from build123d import *

# Parameters (mm, degrees)
SKETCH_1_W          = 15
SKETCH_1_H          = 15.5
SKETCH_1_R          = 2.55
SKETCH_1_R_2        = 3.05
EXTRUDE_1_DEPTH     = 2.5
CUT_EXTRUDE_START   = 2.5
SKETCH_1_4_R        = 0.9
CUT_EXTRUDE_2_DEPTH = 1
SKETCH_1_5_R        = 0.7
CUT_EXTRUDE_3_DEPTH = 14.747221879


with BuildPart() as part:
    # 草图1 → 凸台-拉伸1 (new body)
    with BuildSketch(Plane(origin=(0, 0, 0), x_dir=(1, 0, 0), z_dir=(0, 1, 0))):
        with Locations((0, -0.25)):
            Rectangle(SKETCH_1_W, SKETCH_1_H)
        with Locations(Location((0, -4.7, 0), (0, 0, 270))):
            Circle(SKETCH_1_R, mode=Mode.SUBTRACT)
        with Locations(Location((0, 3.7, 0), (0, 0, 270))):
            Circle(SKETCH_1_R_2, mode=Mode.SUBTRACT)
    extrude(amount=EXTRUDE_1_DEPTH)

    # 草图1<4> → 切除-拉伸2 (cut)
    with BuildSketch(Plane(origin=(0, 0, 0), x_dir=(1, 0, 0), z_dir=(0, 1, 0)).offset(CUT_EXTRUDE_START)):
        with Locations(Location((-6, -6.5, 0), (0, 0, 90))):
            Circle(SKETCH_1_4_R)
        with Locations(Location((6, 3.5, 0), (0, 0, 90))):
            Circle(SKETCH_1_4_R)
        with Locations(Location((-6, 3.5, 0), (0, 0, 90))):
            Circle(SKETCH_1_4_R)
        with Locations(Location((6, -6.5, 0), (0, 0, 90))):
            Circle(SKETCH_1_4_R)
    extrude(amount=-CUT_EXTRUDE_2_DEPTH, mode=Mode.SUBTRACT)

    # 草图1<5> → 切除-拉伸3 (cut, through all)
    with BuildSketch(Plane(origin=(0, 0, 0), x_dir=(1, 0, 0), z_dir=(0, 1, 0)).offset(CUT_EXTRUDE_START)):
        with Locations(Location((-6, -6.5, 0), (0, 0, 90))):
            Circle(SKETCH_1_5_R)
        with Locations(Location((6, 3.5, 0), (0, 0, 90))):
            Circle(SKETCH_1_5_R)
        with Locations(Location((-6, 3.5, 0), (0, 0, 90))):
            Circle(SKETCH_1_5_R)
        with Locations(Location((6, -6.5, 0), (0, 0, 90))):
            Circle(SKETCH_1_5_R)
    extrude(amount=-CUT_EXTRUDE_3_DEPTH, mode=Mode.SUBTRACT)


solid = part.part
Model file for the job. Use its own axes, mm. A direction names the side the tool comes from. Give positions to 0.01 mm unless a question says otherwise; leave off trailing zeros. Loops run counter-clockwise (first coordinate to the right, second up) from the corner with the lowest first, then second, coordinate; pieces in that order, holes last. Notation, with made-up numbers: (-17, 68) -> (-11, 68) arc R19 cw to (-11, 93) -> close; hole circle Ø7 at (27.5, 45.25). An arc over 180 degrees is marked (long way). Use a Markdown table: item, result. Add a question column.
(1) Drop flat-ended pins along their axis: pin 1 Ø1.1 at (x, z) = (6, 6.5) entering from +Y; pin 2 Ø6.5 at (x, z) = (0, 4.7) entering from -Y; pin 3 Ø0.5 at (x, z) = (5.5, -3.5) entering from +Y. Give the stop position or say it passes through.
(2) Tool access for faces 1 (the flat face through (0, 1, -7.5)), 2 (the cylindrical face through (-6.89, 2.01, 6.62)): list every direction of +Z, -Z, +X, -X, +Y, -Y with a clear straight run to the whole face (end or side of a thin tool).
(3) Slice it at D-D on z = -3.7. List the corners of the cut face in (x, y).
(4) Slice it at A-A on x = -6. List the corners of the cut face in (y, z), and give its area (4 significant figures).
(5) Mould opens along X. For faces 3 (the flat face through (-7.5, 1, 0)), 4 (the flat face through (0, 0, 0)), 5 (the cylindrical face through (-6.694, 0.76, -3.409)) say: +X half, -X half, draft (parallel to the pull), parting line (faces both ways), or undercut.
(6) Wall check: line 1 along Z through (x, y) = (-0.25, 1); line 2 along X through (y, z) = (1, 4.7); line 3 along Z through (x, y) = (1.5, 1.7). Give the ranges that are in metal, low to high.
(7) Slice it at B-B on z = 4.7. List the corners of the cut face in (x, y).
(8) Slice it at C-C on y = 2.3. List the corners of the cut face in (x, z), and give its area (3 significant figures).
Filled sheet:
| question | item | result |
|---|---|---|
| 1 | pin 1 | through |
| 1 | pin 2 | y = 0 |
| 1 | pin 3 | y = 1.5 |
| 2 | face 1 | -Z, +X, -X, +Y, -Y |
| 2 | face 2 | +Y |
| 3 | outline | (-7.5, 0) -> (-6.67, 0) -> (-6.67, 1.5) -> (-6.88, 1.5) -> (-6.88, 2.5) -> (-7.5, 2.5) -> close; (-5.33, 0) -> (-3.05, 0) -> (-3.05, 2.5) -> (-5.12, 2.5) -> (-5.12, 1.5) -> (-5.33, 1.5) -> close; (3.05, 0) -> (5.33, 0) -> (5.33, 1.5) -> (5.12, 1.5) -> (5.12, 2.5) -> (3.05, 2.5) -> close; (6.67, 0) -> (7.5, 0) -> (7.5, 2.5) -> (6.88, 2.5) -> (6.88, 1.5) -> (6.67, 1.5) -> close |
| 4 | outline | (0, -7.5) -> (2.5, -7.5) -> (2.5, -4.4) -> (1.5, -4.4) -> (1.5, -4.2) -> (0, -4.2) -> close; (0, -2.8) -> (1.5, -2.8) -> (1.5, -2.6) -> (2.5, -2.6) -> (2.5, 5.6) -> (1.5, 5.6) -> (1.5, 5.8) -> (0, 5.8) -> close; (0, 7.2) -> (1.5, 7.2) -> (1.5, 7.4) -> (2.5, 7.4) -> (2.5, 8) -> (0, 8) -> close |
| 4 | area | 30.95 mm2 |
| 5 | face 3 | -X half |
| 5 | face 4 | draft |
| 5 | face 5 | undercut |
| 6 | line 1 | -7.5 to -6.74, -0.66 to 2.16, 7.24 to 8 |
| 6 | line 2 | -7.5 to -2.55, 2.55 to 7.5 |
| 6 | line 3 | -7.5 to -6.36, -1.04 to 2.64, 6.76 to 8 |
| 7 | outline | (-7.5, 0) -> (-2.55, 0) -> (-2.55, 2.5) -> (-7.5, 2.5) -> close; (2.55, 0) -> (7.5, 0) -> (7.5, 2.5) -> (2.55, 2.5) -> close |
| 8 | outline | (-7.5, -7.5) -> (7.5, -7.5) -> (7.5, 8) -> (-7.5, 8) -> close; hole circle Ø1.8 at (-6, -3.5); hole circle Ø1.8 at (-6, 6.5); hole circle Ø6.1 at (0, -3.7); hole circle Ø5.1 at (0, 4.7); hole circle Ø1.8 at (6, -3.5); hole circle Ø1.8 at (6, 6.5) |
| 8 | area | 173 mm2 |
